The listing builds one solid part. Answer for the finished solid, in the listing's coordinates (mm). A direction names the side the tool comes from. Round coordinates to 2 decimals unless told otherwise and drop trailing zeros. Order: outer loops, then holes, each group sorted by start corner. A loop starts at its lowest first (then second) coordinate and runs counter-clockwise, first axis right, second up. Notation, with made-up numbers: (28.5, 71) - (53.5, 71) arc R35 ccw to (53.5, 104) - close; hole circle Ø5 at (12.5, 6). An arc over 180 degrees is marked (long way). Use CSV: the item, a comma, the result in double quotes. Start each with the question number.
Item 1: Flat-ended cylindrical pins translate along their axes: P1, Ø1.8, axis at x = 11.5, z = 6.5, coming from the +Y side; P2, Ø5.5, axis at x = -36.51, z = 37.2, coming from the +Y side; P3, Ø3, axis at x = -46.2, z = 37.2, coming from the +Y side. Find the tip coordinate at first contact, or state that the pin passes through.
Item 2: Find section B-B, the plane z = 21.5. Give the vertices of the cut face in (x, y).
Item 3: Find section A-A, the plane y = 10. Give the vertices of the cut face in (x, z), plus the area to 3 significant figures.
Item 4: Straight lines are drawn through the part: line 1 along Z through (x, y) = (10, -6.5); line 2 along X through (y, z) = (22, 18.5); line 3 along X through (y, z) = (15.5, 26). For each, find the intervals that lie inside material, in ascending order. Write a range as [from, to].
Item 5: Find section C-C, the plane x = -21.1. Give the vertices of the cut face in (y, z), plus the area to 3 significant figures.
Item 6: Find section D-D, the plane y = 16. Give the vertices of the cut face in (x, z), plus the area to 3 significant figures.
Item 7: Determine the mould class of faces 5 (the flat face through (20, 10, 21)), 6 (the cylindrical face through (-38.258, -11.028, 5.875)), 7 (the flat face through (10, 20, 21)), 8 (the flat face through (-46, 18, 6)) for opening direction Y: +Y half, -Y half, draft (parallel to the pull), parting line (faces both ways), or undercut.
Item 8: For faces 1 (the flat face through (24, 8, 21)), 2 (the flat face through (-47.7, 27.8, 39.8)), 3 (the flat face through (-12, -9, 31)), 4 (the cylindrical face through (9.675, -6.591, 8.277)), determine the directions among +Z, -Z, +X, -X, +Y, -Y from which every point of the face is accessible in a straight line to the end or side of a thin tool.
```python
from build123d import *

# Parameters (mm, degrees)
SKETCH1_W           = 74.2
SKETCH1_H           = 46
BOSS_EXTRUDE1_DEPTH = 43
SKETCH2_R           = 11.5
SKETCH2_R_2         = 1.75
SKETCH2_R_3         = 2.5
CUT_EXTRUDE1_DEPTH  = 20
SKETCH3_R           = 3.1
SKETCH3_R_2         = 1.75
CUT_EXTRUDE2_DEPTH  = 15
CUT_EXTRUDE3_DEPTH  = 2.4
SKETCH5_R           = 2.75
CUT_EXTRUDE4_DEPTH  = 12.4


with BuildPart() as part:
    # Sketch1 → Boss-Extrude1 (new body)
    with BuildSketch(Plane.XY):
        with Locations((-13.1, 10)):
            Rectangle(SKETCH1_W, SKETCH1_H)
        Polygon((0, 0), (20, 0), (20, 20), (0, 20), (0, 29), (-42.2, 29), (-42.2, -9), (0, -9), align=None, mode=Mode.SUBTRACT)
    extrude(amount=BOSS_EXTRUDE1_DEPTH)

    # Sketch2 → Cut-Extrude1 (cut)
    with BuildSketch(Plane.XZ.offset(13)):
        with Locations((-21.1, 21.5)):
            Circle(SKETCH2_R)
        with Locations((-36.509600894, 37.201726029)):
            Circle(SKETCH2_R_2)
        with Locations((-5.690399106, 5.798273971)):
            Circle(SKETCH2_R_2)
        with Locations((-36.509600894, 5.798273971)):
            Circle(SKETCH2_R_2)
        with Locations((-5.690399106, 37.201726029)):
            Circle(SKETCH2_R_2)
        with Locations((10, 37.201726029)):
            Circle(SKETCH2_R_3)
        with Locations((10, 5.798273971)):
            Circle(SKETCH2_R_3)
    extrude(amount=-CUT_EXTRUDE1_DEPTH, mode=Mode.SUBTRACT)

    # Sketch3 → Cut-Extrude2 (cut)
    with BuildSketch(Plane(origin=(0, 33, 0), x_dir=(1, 0, 0), z_dir=(0, 1, 0))):
        with Locations(Location((-36.509600894, -5.798273971, 0), (0, 0, 270))):
            Circle(SKETCH3_R)
        with Locations(Location((-5.690399106, -5.798273971, 0), (0, 0, 270))):
            Circle(SKETCH3_R)
        with Locations(Location((-5.690399106, -37.201726029, 0), (0, 0, 270))):
            Circle(SKETCH3_R)
        with Locations(Location((-36.509600894, -37.201726029, 0), (0, 0, 270))):
            Circle(SKETCH3_R)
        with Locations(Location((-46.2, -5.798273971, 0), (0, 0, 270))):
            Circle(SKETCH3_R_2)
        with Locations(Location((-46.2, -37.201726029, 0), (0, 0, 270))):
            Circle(SKETCH3_R_2)
        with Locations(Location((11.309600894, -5.798273971, 0), (0, 0, 270))):
            Circle(SKETCH3_R_2)
        with Locations(Location((11.309600894, -37.201726029, 0), (0, 0, 270))):
            Circle(SKETCH3_R_2)
    extrude(amount=-CUT_EXTRUDE2_DEPTH, mode=Mode.SUBTRACT)


with BuildPart() as body_2:
    # Split1: the piece on the far side of the plane
    add(part.part)
    split(bisect_by=Plane.ZX.offset(29), keep=Keep.BOTTOM)

    # Sketch4 → Cut-Extrude3 (cut)
    with BuildSketch(Plane(origin=(0, 29, 0), x_dir=(1, 0, 0), z_dir=(0, 1, 0))):
        Polygon((-46.2, -2.334172356), (-49.2, -4.066223163), (-49.2, -7.530324778), (-46.2, -9.262375586), (-43.2, -7.530324778), (-43.2, -4.066223163), align=None)
        Polygon((-43.2, -35.469675222), (-46.2, -33.737624414), (-49.2, -35.469675222), (-49.2, -38.933776837), (-46.2, -40.665827644), (-43.2, -38.933776837), align=None)
        Polygon((14.309600894, -4.066223163), (11.309600894, -2.334172356), (8.309600894, -4.066223163), (8.309600894, -7.530324778), (11.309600894, -9.262375586), (14.309600894, -7.530324778), align=None)
        Polygon((14.309600894, -35.469675222), (11.309600894, -33.737624414), (8.309600894, -35.469675222), (8.309600894, -38.933776837), (11.309600894, -40.665827644), (14.309600894, -38.933776837), align=None)
    extrude(amount=-CUT_EXTRUDE3_DEPTH, mode=Mode.SUBTRACT)

    # Sketch5 → Cut-Extrude4 (cut)
    with BuildSketch(Plane(origin=(24, 0, 0), x_dir=(0, 0, -1), z_dir=(1, 0, 0))):
        with Locations(Location((-35.5, 10, 0), (0, 0, 90))):
            Circle(SKETCH5_R)
        with Locations(Location((-7.5, 10, 0), (0, 0, 90))):
            Circle(SKETCH5_R)
    extrude(amount=-CUT_EXTRUDE4_DEPTH, mode=Mode.SUBTRACT)


with BuildPart() as part_1:
    add(part.part)

    # Split1
    split(bisect_by=Plane.ZX.offset(29), keep=Keep.TOP)


solid = body_2.part
```
Worked out:
1,P1,"stops at y = 0"
1,P2,"stops at y = -9"
1,P3,"stops at y = 18"
2,outline,"(-50.2, -13) - (-32.6, -13) - (-32.6, -9) - (-42.2, -9) - (-42.2, 29) - (-50.2, 29) - close; (-9.6, -13) - (24, -13) - (24, 29) - (0, 29) - (0, 20) - (20, 20) - (20, 0) - (0, 0) - (0, -9) - (-9.6, -9) - close"
3,outline,"(-50.2, 0) - (-42.2, 0) - (-42.2, 43) - (-50.2, 43) - close; (20, 0) - (24, 0) - (24, 4.75) - (20, 4.75) - close; (20, 10.25) - (24, 10.25) - (24, 32.75) - (20, 32.75) - close; (20, 38.25) - (24, 38.25) - (24, 43) - (20, 43) - close"
3,area,"472 mm²"
4,line 1,"z = [0, 3.3], [8.3, 34.7], [39.7, 43]"
4,line 2,"x = [-50.2, -42.2], [0, 24]"
4,line 3,"x = [-50.2, -42.2], [20, 24]"
5,outline,"(-13, 0) - (-9, 0) - (-9, 10) - (-13, 10) - close; (-13, 33) - (-9, 33) - (-9, 43) - (-13, 43) - close"
5,area,"80.0 mm²"
6,outline,"(-50.2, 0) - (-42.2, 0) - (-42.2, 43) - (-50.2, 43) - close; (20, 0) - (24, 0) - (24, 43) - (20, 43) - close"
6,area,"516 mm²"
7,face 5,"undercut"
7,face 6,"draft"
7,face 7,"undercut"
7,face 8,"+Y half"
8,face 1,"+Z, -Z, +X, +Y, -Y"
8,face 2,"+Y"
8,face 3,"+Z, -Z, +Y"
8,face 4,"-Y"
